from build123d import *

# Parameters (mm, degrees)
F0_R     = 42.3758659095
F0_R_2   = 38.1
F0_W     = 50.8
F0_H     = 50.8
F1_DEPTH = 12.7
F2_R     = 38.1
F2_W     = 50.8
F2_H     = 50.8
F3_DEPTH = 57.15
F4_R     = 63.5
F4_R_2   = 38.1
F4_W     = 50.8
F4_H     = 50.8
F5_DEPTH = 25.4
F6_R     = 6.35
F7_DEPTH = 38.1
F8_R     = 5.08


with BuildPart() as f1:
    # F0 (on Front) → F1 (new body)
    with BuildSketch(Plane.XZ):
        Circle(F0_R)
        Circle(F0_R_2, mode=Mode.SUBTRACT)
        Circle(F0_R_2)
        Rectangle(F0_W, F0_H, mode=Mode.SUBTRACT)
    extrude(amount=F1_DEPTH)

    # F2 (on face) → F3 (join)
    with BuildSketch(Plane(origin=(0, 0, 0), x_dir=(-1, 0, 0), z_dir=(0, 1, 0))):
        Circle(F2_R)
        Rectangle(F2_W, F2_H, mode=Mode.SUBTRACT)
    extrude(amount=F3_DEPTH)

    # F4 (on face) → F5 (join)
    with BuildSketch(Plane(origin=(0, 57.15, 0), x_dir=(-1, 0, 0), z_dir=(0, 1, 0))):
        Circle(F4_R)
        Circle(F4_R_2, mode=Mode.SUBTRACT)
        Circle(F4_R_2)
        Rectangle(F4_W, F4_H, mode=Mode.SUBTRACT)
    extrude(amount=F5_DEPTH)

    # F6 (on face) → F7 (cut)
    with BuildSketch(Plane(origin=(0, 82.55, 0), x_dir=(-1, 0, 0), z_dir=(0, 1, 0))):
        with Locations((0, -50.8)):
            Circle(F6_R)
        with Locations((-50.8, 0)):
            Circle(F6_R)
        with Locations((0, 50.8)):
            Circle(F6_R)
        with Locations((50.8, 0)):
            Circle(F6_R)
    extrude(amount=-F7_DEPTH, mode=Mode.SUBTRACT)

    # F8
    f8_edges = [f1.edges().sort_by_distance(p)[0] for p in [
        (-42.375866, -12.7, 0),
    ]]
    fillet(f8_edges, radius=F8_R)


solid = f1.part
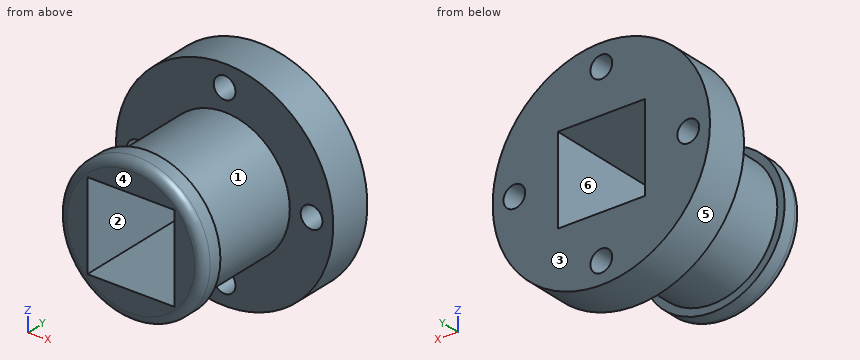
Geometry check sheet. Reference: the model listing, model coordinates, mm. Face numbers are marked on the shaded views. A direction names the side the tool comes from. Round coordinates to 2 decimals unless told otherwise and drop trailing zeros. Order: outer loops, then holes, each group sorted by start corner. A loop starts at its lowest first (then second) coordinate and runs counter-clockwise, first axis right, second up. Notation, with made-up numbers: (-34, 81) -> (-30, 81) arc R19 ccw to (-30, 106) -> close; hole circle Ø11 at (-16.5, 23.5). An arc over 180 degrees is marked (long way). Use one line per item in the form item = value.
1. Cross-section at D-D, the plane z = 50.8. Enter the section's corners in (x, y).
Working result:
outline = (-38.1, 57.15) -> (-6.35, 57.15) -> (-6.35, 82.55) -> (-38.1, 82.55) -> close; (6.35, 57.15) -> (38.1, 57.15) -> (38.1, 82.55) -> (6.35, 82.55) -> close
2. Mould release check, pull along Z, two halves, no side actions. Record for the marked faces 4, 5 and 6: pulls with the +Z half, pulls with the -Z half, needs draft (parallel to the pull), parting line crosses it, or undercut.
Working result:
face_4 = needs draft
face_5 = parting line crosses it
face_6 = undercut
3. Cross-section at B-B, the plane x = 0. Enter the section's corners in (y, z).
Working result:
outline = (-12.7, -37.3) arc R5.08 ccw to (-7.62, -42.38) -> (0, -42.38) -> (0, -38.1) -> (57.15, -38.1) -> (57.15, -44.45) -> (82.55, -44.45) -> (82.55, -25.4) -> (-12.7, -25.4) -> close; (-12.7, 25.4) -> (82.55, 25.4) -> (82.55, 44.45) -> (57.15, 44.45) -> (57.15, 38.1) -> (0, 38.1) -> (0, 42.38) -> (-7.62, 42.38) arc R5.08 ccw to (-12.7, 37.3) -> close; (57.15, -63.5) -> (82.55, -63.5) -> (82.55, -57.15) -> (57.15, -57.15) -> close; (57.15, 57.15) -> (82.55, 57.15) -> (82.55, 63.5) -> (57.15, 63.5) -> close
4. Set-up check for the marked faces 1, 2 and 3: record each of +Z, -Z, +X, -X, +Y, -Y from which the full face is reachable in a straight line by a thin tool's end or side.
Working result:
face_1 = none
face_2 = +Y, -Y
face_3 = +Z, -Z, +X, -X, +Y
5. Scan lines: line 1 along Z through (x, y) = (0, 71.5); line 2 along Y through (x, z) = (-20, -47.5); line 3 along Z through (x, y) = (-23.5, 25). Record each from-to range of solid material in increasing order. Write a range as from..to.
Working result:
line_1 = -63.5..-57.15, -44.45..-25.4, 25.4..44.45, 57.15..63.5
line_2 = 57.15..82.55
line_3 = -29.99..-25.4, 25.4..29.99
6. Cross-section at C-C, the plane y = 28. Enter the section's corners in (x, z).
Working result:
outline = circle Ø76.2 at (0, 0); hole (-25.4, -25.4) -> (25.4, -25.4) -> (25.4, 25.4) -> (-25.4, 25.4) -> close
7. Cross-section at A-A, the plane z = 0. Enter the section's corners in (x, y).
Working result:
outline = (-63.5, 57.15) -> (-57.15, 57.15) -> (-57.15, 82.55) -> (-63.5, 82.55) -> close; (-44.45, 57.15) -> (-38.1, 57.15) -> (-38.1, 0) -> (-42.38, 0) -> (-42.38, -7.62) arc R5.08 ccw to (-37.3, -12.7) -> (-25.4, -12.7) -> (-25.4, 82.55) -> (-44.45, 82.55) -> close; (25.4, -12.7) -> (37.3, -12.7) arc R5.08 ccw to (42.38, -7.62) -> (42.38, 0) -> (38.1, 0) -> (38.1, 57.15) -> (44.45, 57.15) -> (44.45, 82.55) -> (25.4, 82.55) -> close; (57.15, 57.15) -> (63.5, 57.15) -> (63.5, 82.55) -> (57.15, 82.55) -> close
8. Go/stop test with flat-tipped pins: pin 1 (8 mm diameter, centred on y = 29, z = -34.5, fed in from -X); pin 2 (5 mm diameter, centred on y = 43, z = -22.5, fed in from +X); pin 3 (4 mm diameter, centred on x = 44.5, y = 58.5, fed in from +Z); pin 4 (12 mm diameter, centred on x = -8.5, z = -15, fed in from -Y). Record where each tip stops, or that it passes through.
Working result:
pin_1 = -22.83
pin_2 = 32.43
pin_3 = 47.18
pin_4 = through
